Geometry check sheet. Reference: the model listing, model coordinates, mm. A direction names the side the tool comes from. Give positions to 0.01 mm unless a question says otherwise; leave off trailing zeros. Loops run counter-clockwise (first coordinate to the right, second up) from the corner with the lowest first, then second, coordinate; pieces in that order, holes last. Notation, with made-up numbers: (72, 38) -> (125, 38) arc R25 ccw to (125, 65) -> close; hole circle Ø9 at (58.25, -27). An arc over 180 degrees is marked (long way). Write item = value, one per line. Start each with the question number.
```python
from build123d import *

# Parameters (mm, degrees)
SKETCH_1_W               = 20
SKETCH_1_H               = 20
EXTRUDE_1_DEPTH          = 15
SKETCH_1_5_W             = 20
SKETCH_1_5_H             = 20
EXTRUDE_2_DEPTH          = 5
PATTERN_LINEAR_1_COUNT   = 5
PATTERN_LINEAR_1_PITCH   = 40
CUT_EXTRUDE_1_DEPTH      = 181.900525151
CUT_EXTRUDE_1_DEPTH_BACK = 181.900525151
SKETCH_2_W               = 20
SKETCH_2_H               = 20
SKETCH_3_R               = 5
CUT_EXTRUDE_2_DEPTH      = 162.554944214
SKETCH_4_R               = 5
CUT_EXTRUDE_3_DEPTH      = 15
SKETCH_5_R               = 4
CUT_EXTRUDE_4_DEPTH      = 162.554944214
CHAMFER_1_SIZE           = 2
CHAMFER_2_SIZE           = 2
SKETCH_6_R               = 7
CUT_EXTRUDE_5_DEPTH      = 4


with BuildPart() as part:
    # Sketch 1 → Extrude 1 (new body)
    with BuildSketch(Plane.XY):
        with Locations((0, 10)):
            Rectangle(SKETCH_1_W, SKETCH_1_H)
    extrude(amount=EXTRUDE_1_DEPTH)

    # Sketch 1_5 → Extrude 2 (add)
    with BuildSketch(Plane.XY):
        with Locations((0, 10)):
            Rectangle(SKETCH_1_5_W, SKETCH_1_5_H)
        with Locations((0, -10)):
            Rectangle(SKETCH_1_5_W, SKETCH_1_5_H)
    extrude(amount=-EXTRUDE_2_DEPTH)


with BuildPart() as pattern_linear_1_1:
    # Pattern Linear 1: pattern copy
    add(part.part.moved(Location(Vector(0, -1, 0) * (1 * PATTERN_LINEAR_1_PITCH))))

    # Sketch 4 → Cut-Extrude 3 (cut)
    with BuildSketch(Plane.XY.offset(15)):
        with Locations((0, -30)):
            Circle(SKETCH_4_R)
    extrude(amount=-CUT_EXTRUDE_3_DEPTH, mode=Mode.SUBTRACT)


with BuildPart() as pattern_linear_1_2:
    # Pattern Linear 1: pattern copy
    add(part.part.moved(Location(Vector(0, -1, 0) * (2 * PATTERN_LINEAR_1_PITCH))))


with BuildPart() as pattern_linear_1_3:
    # Pattern Linear 1: pattern copy
    add(part.part.moved(Location(Vector(0, -1, 0) * (3 * PATTERN_LINEAR_1_PITCH))))


with BuildPart() as pattern_linear_1_4:
    # Pattern Linear 1: pattern copy
    add(part.part.moved(Location(Vector(0, -1, 0) * (4 * PATTERN_LINEAR_1_PITCH))))

    # Sketch 2 → Cut-Extrude 1 (cut, two sides: drawn at the far end of the back side and taken through both)
    with BuildSketch(Plane.XY.offset(-CUT_EXTRUDE_1_DEPTH_BACK)):
        with Locations((0, -170)):
            Rectangle(SKETCH_2_W, SKETCH_2_H)
    extrude(amount=CUT_EXTRUDE_1_DEPTH + CUT_EXTRUDE_1_DEPTH_BACK, mode=Mode.SUBTRACT)


with BuildPart() as part_1:
    add(part.part)

    # Sketch 3 → Cut-Extrude 2 (cut, through all)
    with BuildSketch(Plane.XY.offset(15)):
        with Locations((0, 10)):
            Circle(SKETCH_3_R)
    extrude(amount=-CUT_EXTRUDE_2_DEPTH, mode=Mode.SUBTRACT)


with BuildPart() as cut_extrude_4_tool:
    # Sketch 5 → Cut-Extrude 4 (new, through all)
    with BuildSketch(Plane.XY.offset(15)):
        with Locations((0, -70)):
            Circle(SKETCH_5_R)
        with Locations((0, -110)):
            Circle(SKETCH_5_R)
        with Locations((0, -150)):
            Circle(SKETCH_5_R)
    extrude(amount=-CUT_EXTRUDE_4_DEPTH)


with BuildPart() as pattern_linear_1_2_1:
    add(pattern_linear_1_2.part)

    # Cut-Extrude 4: cut by cut_extrude_4_tool
    add(cut_extrude_4_tool.part, mode=Mode.SUBTRACT)

    # Chamfer 1
    chamfer_1_edges = [pattern_linear_1_2_1.edges().sort_by_distance(p)[0] for p in [
        (-4, -70, 15),
    ]]
    chamfer(chamfer_1_edges, length=CHAMFER_1_SIZE)


with BuildPart() as pattern_linear_1_3_1:
    add(pattern_linear_1_3.part)

    # Cut-Extrude 4: cut by cut_extrude_4_tool
    add(cut_extrude_4_tool.part, mode=Mode.SUBTRACT)

    # Chamfer 2
    chamfer_2_edges = [pattern_linear_1_3_1.edges().sort_by_distance(p)[0] for p in [
        (-4, -110, 15),
    ]]
    chamfer(chamfer_2_edges, length=CHAMFER_2_SIZE)


with BuildPart() as pattern_linear_1_4_1:
    add(pattern_linear_1_4.part)

    # Cut-Extrude 4: cut by cut_extrude_4_tool
    add(cut_extrude_4_tool.part, mode=Mode.SUBTRACT)

    # Sketch 6 → Cut-Extrude 5 (cut)
    with BuildSketch(Plane.XY.offset(15)):
        with Locations((0, -150)):
            Circle(SKETCH_6_R)
    extrude(amount=-CUT_EXTRUDE_5_DEPTH, mode=Mode.SUBTRACT)


with BuildPart() as part_2:
    add(part_1.part)

    # Combine 1: union Pattern Linear 1_1, Pattern Linear 1_2, Pattern Linear 1_3, Pattern Linear 1_4
    add(pattern_linear_1_1.part)
    add(pattern_linear_1_2_1.part)
    add(pattern_linear_1_3_1.part)
    add(pattern_linear_1_4_1.part)


solid = part_2.part
```
1) Tool access check on faces 5 (the flat face through (0, 20, 5)), 6 (the flat face through (0, -50, 0)), 7 (the flat face through (0, -30, 0)). Record the directions out of +Z, -Z, +X, -X, +Y, -Y that give a thin tool (end or side, any length) a straight path to the whole face; none if there is none.
2) Section check B-B (y = 10). Enter the section's corners in (x, z), plus the area to 3 significant figures.
3) Depth check by flat-ended pin: pin 1 Ø11 at (x, y) = (0, -150) entering from -Z. Enter the tip coordinate at first touch or a pass-through.
4) Section check A-A (z = 2.5). Give the number of separate pieces and of enclosed holes in the cut face, plus the area to 3 significant figures.
5) Thickness scan on line 1 (Y direction, x = -7.5, z = 9.5); line 2 (Y direction, x = 3.5, z = -3.25); line 3 (Z direction, x = -7.25, y = -87). Record the ranges inside material, lowest first.
6) Draft check along X on faces 1 (the cylindrical face through (-1.08, -34.88, 7.6)), 2 (the cylindrical face through (-0.521, -146.034, 3.112)), 3 (the flat face through (0, -120, 7)), 4 (the flat face through (-10, -69, 3)). Enter one of: released by +X, released by -X, zero draft, split by the parting line, or undercut.
7) Section check C-C (y = -30). Enter the section's corners in (x, z), plus the area to 3 significant figures.
Check result:
q1.face_5 = +Z, -Z, +X, -X, +Y
q1.face_6 = +Z, +X, -X
q1.face_7 = +Z
q2.outline = (-10, -5) -> (-5, -5) -> (-5, 15) -> (-10, 15) -> close; (5, -5) -> (10, -5) -> (10, 15) -> (5, 15) -> close
q2.area = 200 mm2
q3.pin_1 = -5
q4.separate_pieces = 5
q4.enclosed_holes = 5
q4.area = 1,690 mm2
q5.line_1 = -160 to -140, -120 to -100, -80 to -60, -40 to -20, 0 to 20
q5.line_2 = -160 to -151.94, -148.06 to -111.94, -108.06 to -71.94, -68.06 to 6.43, 13.57 to 20
q5.line_3 = -5 to 0
q6.face_1 = undercut
q6.face_2 = undercut
q6.face_3 = zero draft
q6.face_4 = released by -X
q7.outline = (-10, -5) -> (10, -5) -> (10, 15) -> (5, 15) -> (5, 0) -> (-5, 0) -> (-5, 15) -> (-10, 15) -> close
q7.area = 250 mm2
